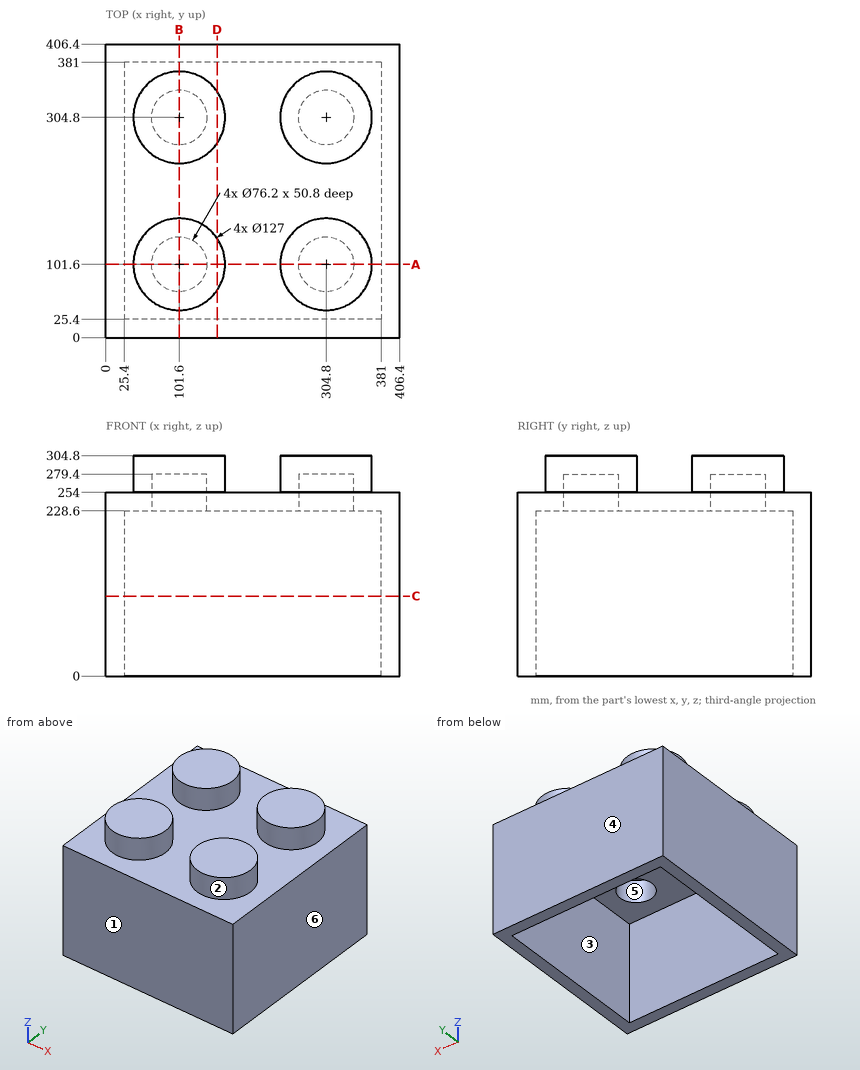
Print and shaded views of the part. All mm, measured from the part's lowest x, y and z. A direction names the side the tool comes from. Give positions to 0.01 mm unless a question says otherwise; leave off trailing zeros. Order: outer loops, then holes, each group sorted by start corner. A loop starts at its lowest first (then second) coordinate and runs counter-clockwise, first axis right, second up. Notation, with made-up numbers: (-11, 7) - (34, 7) arc R15 ccw to (34, 17) - close; hole circle Ø10 at (26, 58.25). An arc over 180 degrees is marked (long way). Use a Markdown table: item, result.
1) Two-plate mould, pull along Y, no slides. Class the marked faces 4, 5 and 6: +Y half, -Y half, draft (parallel to the pull), parting line (faces both ways), or undercut.
Checked values:
| item | result |
|---|---|
| face 4 | +Y half |
| face 5 | undercut |
| face 6 | draft |
2) Flat gauge pins, fed straight in: P1, Ø23, axis at x = 308, y = 313.5, coming from the -Z side; P2, Ø5, axis at x = 235, y = 154, coming from the +Z side; P3, Ø2, axis at x = 253.5, y = 131, coming from the -Z side; P4, Ø8, axis at x = 233.5, z = 259.5, coming from the -Y side. Where does each tip first touch, or does it go through?
Checked values:
| item | result |
|---|---|
| P1 | z = 279.4 |
| P2 | z = 254 |
| P3 | z = 228.6 |
| P4 | through |
3) Saw through at C-C on z = 110.5. List the corners of the cut face in (x, y), plus the area to 3 significant figures.
Checked values:
| item | result |
|---|---|
| outline | (0, 0) - (406.4, 0) - (406.4, 406.4) - (0, 406.4) - close; hole (25.4, 25.4) - (381, 25.4) - (381, 381) - (25.4, 381) - close |
| area | 38,700 mm² |
4) Saw through at A-A on y = 101.6. List the corners of the cut face in (x, z), plus the area to 3 significant figures.
Checked values:
| item | result |
|---|---|
| outline | (0, 0) - (25.4, 0) - (25.4, 228.6) - (63.5, 228.6) - (63.5, 279.4) - (139.7, 279.4) - (139.7, 228.6) - (266.7, 228.6) - (266.7, 279.4) - (342.9, 279.4) - (342.9, 228.6) - (381, 228.6) - (381, 0) - (406.4, 0) - (406.4, 254) - (368.3, 254) - (368.3, 304.8) - (241.3, 304.8) - (241.3, 254) - (165.1, 254) - (165.1, 304.8) - (38.1, 304.8) - (38.1, 254) - (0, 254) - close |
| area | 27,100 mm² |
5) Saw through at D-D on x = 154. List the corners of the cut face in (y, z), plus the area to 3 significant figures.
Checked values:
| item | result |
|---|---|
| outline | (0, 0) - (25.4, 0) - (25.4, 228.6) - (381, 228.6) - (381, 0) - (406.4, 0) - (406.4, 254) - (340.67, 254) - (340.67, 304.8) - (268.93, 304.8) - (268.93, 254) - (137.47, 254) - (137.47, 304.8) - (65.73, 304.8) - (65.73, 254) - (0, 254) - close |
| area | 29,200 mm² |
6) Probe L1, parallel to X at y = 304, z = 239; L2, parallel to Y at x = 304.8, z = 244; L3, parallel to X at y = 365, z = 91.5. List the from-to ranges inside material, lowest first. Write a range as from..to.
Checked values:
| item | result |
|---|---|
| L1 | 0..63.51, 139.69..266.71, 342.89..406.4 |
| L2 | 0..63.5, 139.7..266.7, 342.9..406.4 |
| L3 | 0..25.4, 381..406.4 |
7) 3-axis set-ups, long thin cutter, end or side, ignore diameter. For the marked faces 1, 2 and 3: which of +Z, -Z, +X, -X, +Y, -Y reach the whole face in a straight line?
Checked values:
| item | result |
|---|---|
| face 1 | +Z, -Z, +X, -X, -Y |
| face 2 | +Z |
| face 3 | -Z |
